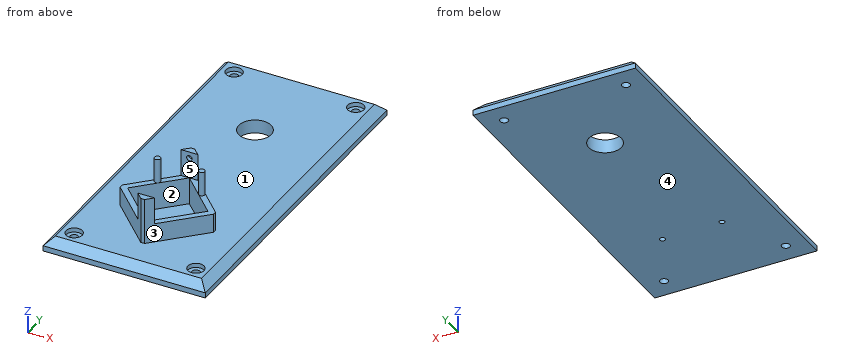
```python
from build123d import *

# Parameters (mm, degrees)
PAD_DEPTH            = 22
POCKET_DEPTH         = 20
POCKET001_DEPTH      = 10
SKETCH003_R          = 1
POCKET002_DEPTH      = 16.25
POCKET002_DEPTH_BACK = -16.25
SKETCH004_R          = 1.1
PAD001_DEPTH         = 9
SKETCH005_R          = 1
POCKET003_DEPTH      = 5
SKETCH006_W          = 60
SKETCH006_H          = 125
PAD002_DEPTH         = 5
CHAMFER_SIZE         = 3
CHAMFER001_SIZE      = 1
SKETCH007_R          = 6
POCKET004_DEPTH      = 5
SKETCH008_R          = 1.5
POCKET005_DEPTH      = 5
SKETCH009_R          = 3
POCKET006_DEPTH      = 1.6


with BuildPart() as part:
    # Sketch → Pad (new body)
    with BuildSketch(Plane.XY):
        Polygon((0, -17.960512), (17.960512, 0), (0, 17.960512), (-17.960512, 0), align=None)
    extrude(amount=PAD_DEPTH)

    # Sketch001 (on Face6 of Pad) → Pocket (cut)
    with BuildSketch(Plane.XY.offset(22)):
        Polygon((0, 14.849242), (-14.849242, 0), (0, -14.849242), (14.849242, 0), align=None)
    extrude(amount=-POCKET_DEPTH, mode=Mode.SUBTRACT)

    # Sketch002 (on Face5 of Pocket) → Pocket001 (cut)
    with BuildSketch(Plane.XY.offset(22)):
        Polygon((-3.11127, 14.849242), (-17.960512, 0), (-3.11127, -14.849242), (0, -14.849242), (-14.849242, 0), (0, 14.849242), align=None)
    pocket001 = extrude(amount=-POCKET001_DEPTH, mode=Mode.SUBTRACT)

    # Mirrored: Pocket001 across YZ
    add(pocket001.mirror(Plane.YZ), mode=Mode.SUBTRACT)

    # Sketch003 → Pocket002 (cut, two sides)
    with BuildSketch(Plane.XZ) as pocket002_sk:
        with Locations((0, 19.622342)):
            Circle(SKETCH003_R)
    extrude(amount=-POCKET002_DEPTH, mode=Mode.SUBTRACT)
    extrude(pocket002_sk.sketch, amount=-POCKET002_DEPTH_BACK, mode=Mode.SUBTRACT)

    # Sketch004 (on Face15 of Pocket002) → Pad001 (join)
    with BuildSketch(Plane.XY.offset(12)):
        with Locations((8.202439, 8.202439)):
            Circle(SKETCH004_R)
    pad001 = extrude(amount=PAD001_DEPTH)

    # Mirrored001: Pad001 across YZ
    add(pad001.mirror(Plane.YZ))

    # Sketch005 (on Face21 of Mirrored001) → Pocket003 (cut)
    with BuildSketch(Plane.XY.offset(2)):
        with Locations((-11, 0)):
            Circle(SKETCH005_R)
        with Locations((11, 0)):
            Circle(SKETCH005_R)
    extrude(amount=-POCKET003_DEPTH, mode=Mode.SUBTRACT)

    # Sketch006 (on Face2 of Pocket003) → Pad002 (join)
    with BuildSketch(Plane(origin=(0, 0, 0), x_dir=(1, 0, 0), z_dir=(0, 0, -1))):
        with Locations((0, -32.5)):
            Rectangle(SKETCH006_W, SKETCH006_H)
        Polygon((0, 17.526509), (-17.526509, 0), (0, -17.526509), (17.526509, 0), align=None, mode=Mode.SUBTRACT)
    extrude(amount=-PAD002_DEPTH)

    # Chamfer
    chamfer_edges = [part.edges().sort_by_distance(p)[0] for p in [
        (30, 32.5, 5),
        (0, 95, 5),
        (-30, 32.5, 5),
        (0, -30, 5),
    ]]
    chamfer(chamfer_edges, length=CHAMFER_SIZE)

    # Chamfer001
    chamfer001_edges = [part.edges().sort_by_distance(p)[0] for p in [
        (17.960512, 0, 8.5),
        (0, 17.960512, 13.5),
        (-17.960512, 0, 8.5),
        (0, -17.960512, 13.5),
    ]]
    chamfer(chamfer001_edges, length=CHAMFER001_SIZE)

    # Sketch007 (on Face1 of Chamfer001) → Pocket004 (cut)
    with BuildSketch(Plane.XY.offset(5)):
        with Locations((0, 60)):
            Circle(SKETCH007_R)
    extrude(amount=-POCKET004_DEPTH, mode=Mode.SUBTRACT)

    # Sketch008 (on Face1 of Pocket004) → Pocket005 (cut)
    with BuildSketch(Plane.XY.offset(5)):
        with Locations((-22.5, 87.5)):
            Circle(SKETCH008_R)
        with Locations((22.5, 87.5)):
            Circle(SKETCH008_R)
        with Locations((22.5, -22.5)):
            Circle(SKETCH008_R)
        with Locations((-22.5, -22.5)):
            Circle(SKETCH008_R)
    extrude(amount=-POCKET005_DEPTH, mode=Mode.SUBTRACT)

    # Sketch009 (on Face1 of Pocket005) → Pocket006 (cut)
    with BuildSketch(Plane.XY.offset(5)):
        with Locations((-22.5, 87.5)):
            Circle(SKETCH009_R)
        with Locations((22.5, 87.5)):
            Circle(SKETCH009_R)
        with Locations((-22.5, -22.5)):
            Circle(SKETCH009_R)
        with Locations((22.5, -22.5)):
            Circle(SKETCH009_R)
    extrude(amount=-POCKET006_DEPTH, mode=Mode.SUBTRACT)


solid = part.part
```
Work out the finished part from the listing and answer in its coordinate system (mm). Face numbers are marked on the shaded views. A direction names the side the tool comes from. Coordinates: 2 decimals unless noted, no trailing zeros. Write each loop counter-clockwise with the first axis right and the second up, starting at its lowest first coordinate (ties: lowest second). Pieces come first, ordered by that corner, then holes.
Q1. A cutting plane is placed at A-A, the plane y = -22.5. Give the vertices of the cut face in (x, z), then the cut area to 3 significant figures.
Q2. A cutting plane is placed at B-B, the plane x = 22.5. Give the vertices of the cut face in (y, z), then the cut area to 3 significant figures.
Q3. Which of the six approach directions +Z, -Z, +X, -X, +Y, -Y give full straight-line access (tool end or side, diameter ignored) to the marked faces 4 and 5?
Q4. Find the intervals of material crossed by line 1 (X direction, y = 87.5, z = 1.45); line 2 (Z direction, x = 0, y = -15); line 3 (Y direction, x = 22.5, z = 4.6), in increasing order.
Q5. A cutting plane is placed at D-D, the plane y = 63.5. Give the vertices of the cut face in (x, z).
Q6. A cutting plane is placed at C-C, the plane z = 13.75. Give the vertices of the cut face in (x, y).
Q7. Each of these flat-tipped pins is pushed along its axis until it touches: pin 1 Ø3.5 at (x, y) = (22.5, 87.5) entering from -Z; pin 2 Ø9 at (x, y) = (4, -1) entering from +Z; pin 3 Ø4 at (x, y) = (11, 21) entering from +Z; pin 4 Ø6 at (x, z) = (-16.5, 17) entering from -Y. Where does it stop, or does it pass through?
Q8. Determine the mould class of the marked faces 1, 2 and 3 for opening direction Y: released by +Y, released by -Y, zero draft, split by the parting line, or undercut.
Findings below:
1. outline: (-30, 0) - (-24, 0) - (-24, 3.4) - (-25.5, 3.4) - (-25.5, 5) - (-27, 5) - (-30, 2) - close; (-21, 0) - (21, 0) - (21, 3.4) - (19.5, 3.4) - (19.5, 5) - (-19.5, 5) - (-19.5, 3.4) - (-21, 3.4) - close; (24, 0) - (30, 0) - (30, 2) - (27, 5) - (25.5, 5) - (25.5, 3.4) - (24, 3.4) - close
1. area: 251 mm2
2. outline: (-30, 0) - (-24, 0) - (-24, 3.4) - (-25.5, 3.4) - (-25.5, 5) - (-27, 5) - (-30, 2) - close; (-21, 0) - (86, 0) - (86, 3.4) - (84.5, 3.4) - (84.5, 5) - (-19.5, 5) - (-19.5, 3.4) - (-21, 3.4) - close; (89, 0) - (95, 0) - (95, 2) - (92, 5) - (90.5, 5) - (90.5, 3.4) - (89, 3.4) - close
2. area: 576 mm2
3. face 4: -Z, +X, -X, +Y, -Y
3. face 5: +Z, +X, -X
4. line 1: x = -30 to -24, -21 to 21, 24 to 30
4. line 2: z = 0 to 18.62, 20.62 to 22
4. line 3: y = -27.4 to -25.5, -19.5 to 84.5, 90.5 to 92.4
5. outline: (-30, 0) - (-4.87, 0) - (-4.87, 5) - (-27, 5) - (-30, 2) - close; (4.87, 0) - (30, 0) - (30, 2) - (27, 5) - (4.87, 5) - close
6. outline: circle Ø2.2 at (-8.2, 8.2); (-3.11, -14.85) - (-0.71, -17.25) - (0.71, -17.25) - (3.11, -14.85) - close; (-3.11, 14.85) - (3.11, 14.85) - (0.71, 17.25) - (-0.71, 17.25) - close; circle Ø2.2 at (8.2, 8.2)
7. pin 1: stops at z = 0
7. pin 2: stops at z = 2
7. pin 3: stops at z = 5
7. pin 4: passes through
8. face 1: zero draft
8. face 2: undercut
8. face 3: released by -Y
